Geometry: final body of the model. Coordinates: model frame, mm. Face numbers are marked on the shaded views. A direction names the side the tool comes from. Give positions to 0.01 mm unless a question says otherwise; leave off trailing zeros. Order: outer loops, then holes, each group sorted by start corner. A loop starts at its lowest first (then second) coordinate and runs counter-clockwise, first axis right, second up. Notation, with made-up numbers: M 89.25,40.25 L 139.25,40.25 A19 cw 139.25,72.25 Z; hole C -31.5,78 d10. An arc over 180 degrees is marked long. Write item = value, one per line. Start each with the question number.
from build123d import *

# Parameters (mm, degrees)
CUT_EXTRUDE_1_DEPTH    = 6
CUT_EXTRUDE_2_DEPTH    = 5.5
CHAMFER_1_SIZE         = 2
HOLE_WIZARD_M6_1_D     = 5
HOLE_WIZARD_M6_1_DEPTH = 17
HOLE_WIZARD_M6_1_TIP   = 1.502151548


with BuildPart() as part:
    # 草图1 → 旋转1 (revolve)
    with BuildSketch(Plane.XY, mode=Mode.PRIVATE) as revolve_1_sk:
        Polygon((-76.99110035, 0), (188.00889965, 0), (188.00889965, 22.5), (123.00889965, 22.5), (123.00889965, 25), (61.00889965, 25), (61.00889965, 27.5), (21.00889965, 27.5), (21.00889965, 29), (-34.99110035, 29), (-34.99110035, 31), (-42.99110035, 31), (-42.99110035, 27.5), (-76.99110035, 27.5), align=None)
    revolve(revolve_1_sk.sketch.rotate(Axis((-104.076979444, 0, 0), (1, 0, 0)), 90), axis=Axis((-104.076979444, 0, 0), (1, 0, 0)))

    # 草图2 → 切除-拉伸1 (cut)
    with BuildSketch(Plane(origin=(0, 29, 0), x_dir=(-1, 0, 0), z_dir=(0, 1, 0))):
        with BuildLine():
            Line((23.99110035, -8), (-10.00889965, -8))
            ThreePointArc((-10.00889965, -8), (-18.00889965, 0), (-10.00889965, 8))
            Line((-10.00889965, 8), (23.99110035, 8))
            ThreePointArc((23.99110035, 8), (31.99110035, 0), (23.99110035, -8))
        make_face()
    extrude(amount=-CUT_EXTRUDE_1_DEPTH, mode=Mode.SUBTRACT)

    # 草图3 → 切除-拉伸2 (cut)
    with BuildSketch(Plane(origin=(0, 22.5, 0), x_dir=(-1, 0, 0), z_dir=(0, 1, 0))):
        with BuildLine():
            Line((-176.50889965, 7), (-134.50889965, 7))
            ThreePointArc((-134.50889965, 7), (-129.559152182, 4.949747468), (-127.50889965, 0))
            ThreePointArc((-127.50889965, 0), (-129.559152182, -4.949747468), (-134.50889965, -7))
            Line((-134.50889965, -7), (-176.50889965, -7))
            ThreePointArc((-176.50889965, -7), (-181.458647118, -4.949747468), (-183.50889965, 0))
            ThreePointArc((-183.50889965, 0), (-181.458647118, 4.949747468), (-176.50889965, 7))
        make_face()
    extrude(amount=-CUT_EXTRUDE_2_DEPTH, mode=Mode.SUBTRACT)

    # 倒角1
    chamfer_1_edges = [part.edges().sort_by_distance(p)[0] for p in [
        (188.00889965, 0, -22.5),
        (-76.99110035, 0, -27.5),
    ]]
    chamfer(chamfer_1_edges, length=CHAMFER_1_SIZE)

    # M6 螺纹孔1
    with Locations(Plane(origin=(188.00889965, 0, 0), x_dir=(0, 0, -1), z_dir=(1, 0, 0))):
        with Locations((0, 10), (0, -10)):
            Hole(HOLE_WIZARD_M6_1_D / 2, depth=HOLE_WIZARD_M6_1_DEPTH)
            with Locations((0, 0, -(HOLE_WIZARD_M6_1_DEPTH + HOLE_WIZARD_M6_1_TIP / 2))):  # 118° drill point
                Cone(0, HOLE_WIZARD_M6_1_D / 2, HOLE_WIZARD_M6_1_TIP, mode=Mode.SUBTRACT)


solid = part.part
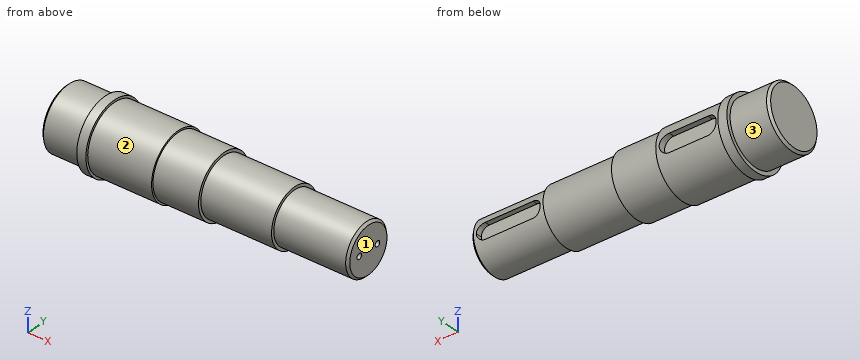
1) Cut plane A-A (y = 0). Return loops of the section in (x, z), plus the area to 3 significant figures.
2) Access query for the marked faces 1, 2 and 3. Directions: +Z, -Z, +X, -X, +Y, -Y. A direction counts if a zero-diameter tool reaches every point of the face in a straight line with its end or side. Return the directions, or none.
3) Ray query, L1, parallel to Y at x = 181, z = 0; L2, parallel to Z at x = 33, y = -1; L3, parallel to Z at x = 183, y = 10. Return the intervals inside material, ascending.
4) Pin query (flat end, axial travel): pin 1 Ø1.5 at (x, y) = (-14.5, 25.5) entering from +Z; pin 2 Ø8 at (x, z) = (5, -0.5) entering from +Y; pin 3 Ø2 at (x, z) = (110.5, -4.5) entering from -Y. Return the tip coordinate at first contact, or that it passes through.
5) Cut plane C-C (x = 87). Return loops of the section in (y, z).
6) Cut plane D-D (x = 167). Return loops of the section in (y, z).
7) Cut plane B-B (x = -14). Return loops of the section in (y, z).
Reply:
q1.outline = M -76.99,-25.5 L -74.99,-27.5 L -42.99,-27.5 L -42.99,-31 L -34.99,-31 L -34.99,-29 L 21.01,-29 L 21.01,-27.5 L 61.01,-27.5 L 61.01,-25 L 123.01,-25 L 123.01,-22.5 L 186.01,-22.5 L 188.01,-20.5 L 188.01,20.5 L 186.01,22.5 L 123.01,22.5 L 123.01,25 L 61.01,25 L 61.01,27.5 L 21.01,27.5 L 21.01,29 L -34.99,29 L -34.99,31 L -42.99,31 L -42.99,27.5 L -74.99,27.5 L -76.99,25.5 Z
q1.area = 13,800 mm²
q2.face_1 = +Z, -Z, +X, +Y, -Y
q2.face_2 = +X
q2.face_3 = -X
q3.L1 = -22.5 to -12.5, -7.5 to 7.5, 12.5 to 17
q3.L2 = -27.48 to 27.48
q3.L3 = -20.16 to -2.5, 2.5 to 20.16
q4.pin_1 = 15.11
q4.pin_2 = 23
q4.pin_3 = -24.75
q5.outline = C 0,0 d50
q6.outline = M 17,-7 L 17,7 L 21.38,7 A22.5 ccw long 21.38,-7 Z
q7.outline = M 23,-8 L 23,8 L 27.87,8 A29 ccw long 27.87,-8 Z
